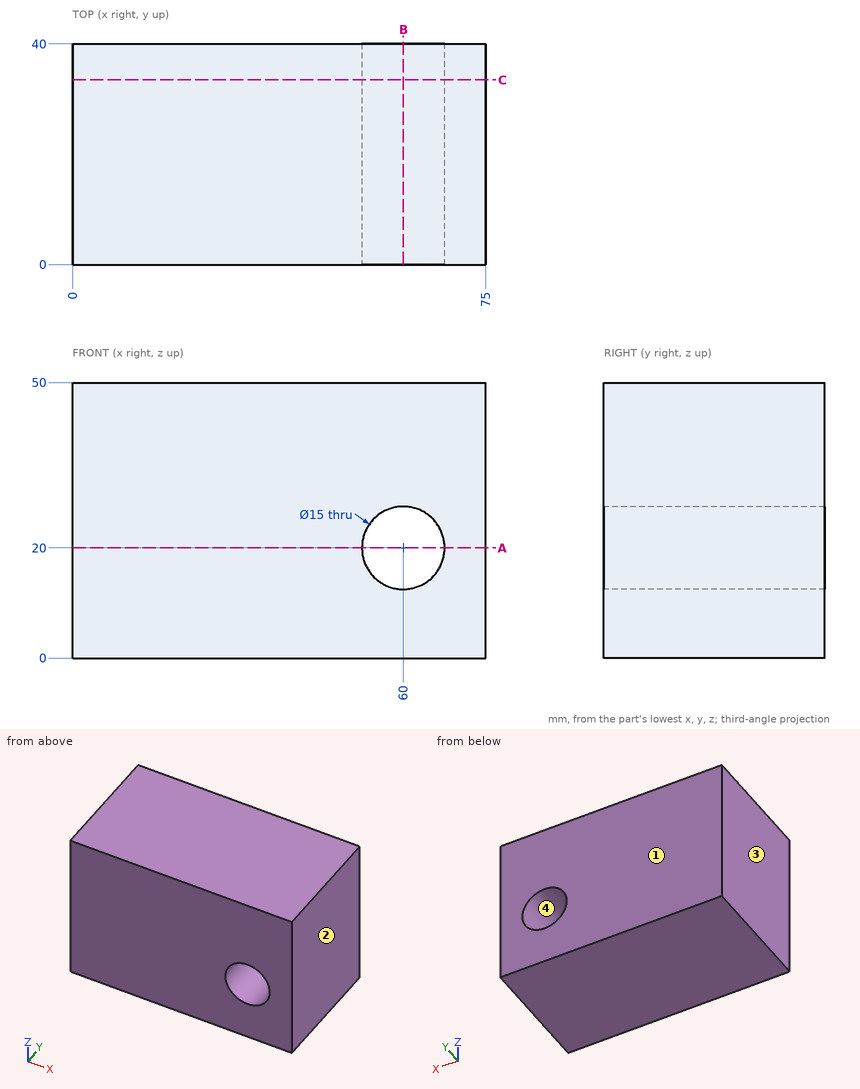
Input: dimensioned drawing with shaded views. Units: mm. Origin: part minimum x, y, z. Coordinates: 2 decimals unless noted, no trailing zeros. Loops run counter-clockwise (first coordinate to the right, second up) from the corner with the lowest first, then second, coordinate; pieces in that order, holes last. Notation, with made-up numbers: M -17,86 L -12,86 A10 ccw -12,104 Z; hole C 41,-0.5 d9. An arc over 180 degrees is marked long. Use a Markdown table: item, result. Add a question column.
1) Section C-C, the plane y = 33.5. Return the cut outline in (x, z), plus the area to 3 significant figures.
2) Draft query along X for the marked faces 1, 2, 3 and 4. Return one class per face: +X half, -X half, draft (parallel to the pull), parting line (faces both ways), or undercut.
3) Section A-A, the plane z = 20. Return the cut outline in (x, y), plus the area to 3 significant figures.
4) Line query: L1, parallel to Z at x = 60, y = 13; L2, parallel to X at y = 16, z = 19.5; L3, parallel to X at y = 25, z = 13.5. Output: solid intervals per line, ascending. Write a range as from..to.
5) Section B-B, the plane x = 60. Return the cut outline in (y, z).
Answer below:
| question | item | result |
|---|---|---|
| 1 | outline | M 0,0 L 75,0 L 75,50 L 0,50 Z; hole C 60,20 d15 |
| 1 | area | 3,570 mm2 |
| 2 | face 1 | draft |
| 2 | face 2 | +X half |
| 2 | face 3 | -X half |
| 2 | face 4 | undercut |
| 3 | outline | M 0,0 L 52.5,0 L 52.5,40 L 0,40 Z; M 67.5,0 L 75,0 L 75,40 L 67.5,40 Z |
| 3 | area | 2,400 mm2 |
| 4 | L1 | 0..12.5, 27.5..50 |
| 4 | L2 | 0..52.52, 67.48..75 |
| 4 | L3 | 0..56.26, 63.74..75 |
| 5 | outline | M 0,0 L 40,0 L 40,12.5 L 0,12.5 Z; M 0,27.5 L 40,27.5 L 40,50 L 0,50 Z |
